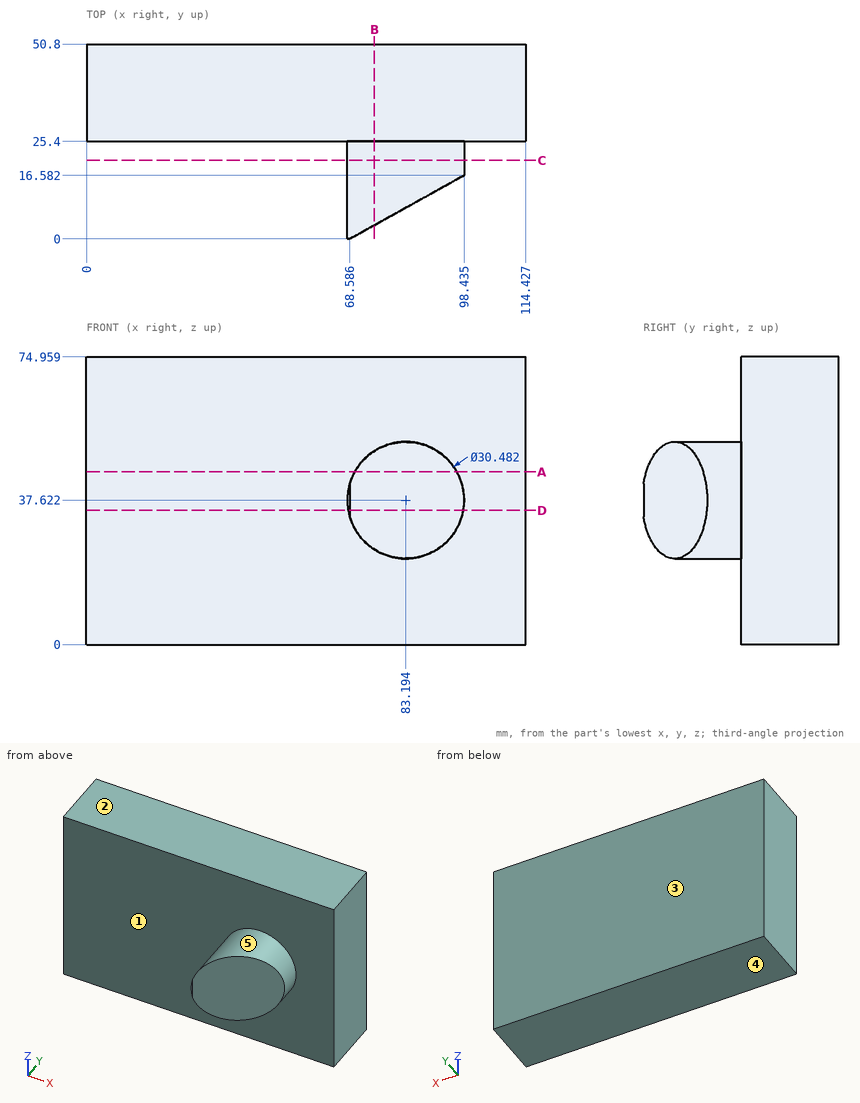
For this review, use the dimensioned drawing (mm, ordinates from the lowest corner) and the shaded views. A direction names the side the tool comes from. Round coordinates to 2 decimals unless told otherwise and drop trailing zeros. Order: outer loops, then holes, each group sorted by start corner. A loop starts at its lowest first (then second) coordinate and runs counter-clockwise, first axis right, second up. Notation, with made-up numbers: (-28, 58.5) -> (5, 58.5) arc R18 cw to (5, 80.5) -> close; hole circle Ø8 at (-0.75, 5). An arc over 180 degrees is marked (long way). Put each result on its own line as item: value.
Q1. Mouldability with a two-part tool opening along Y and no side actions: class the marked faces 1, 2 and 3 as pulls with the +Y half, pulls with the -Y half, needs draft (parallel to the pull), parting line crosses it, or undercut.
Check result:
face 1: pulls with the -Y half
face 2: needs draft
face 3: pulls with the +Y half
Q2. Insertion check: pin 1 Ø12 at (x, y) = (64.5, 10.5) entering from -Z (1 decimal); pin 2 Ø1.5 at (x, y) = (102, 26.5) entering from -Z; pin 3 Ø2 at (x, y) = (86, 21.5) entering from +Z (1 decimal); pin 4 Ø2 at (y, z) = (9.5, 23) entering from +X (1 decimal). Each pin has a flat end and moves straight along its axis. Give the tip position at first contact, or say it passes through.
Check result:
pin 1: z = 29.2
pin 2: z = 0
pin 3: z = 52.8
pin 4: x = 87.5
Q3. Add section A-A on z = 45. Write out the cut boundary in (x, y) (1 decimal).
Check result:
outline: (0, 25.4) -> (69.9, 25.4) -> (69.9, 0.7) -> (96.5, 15.5) -> (96.5, 25.4) -> (114.4, 25.4) -> (114.4, 50.8) -> (0, 50.8) -> close
Q4. Add section D-D on z = 35. Write out the cut boundary in (x, y).
Check result:
outline: (0, 25.4) -> (68.18, 25.4) -> (68.18, 0) -> (68.59, 0) -> (98.21, 16.46) -> (98.21, 25.4) -> (114.43, 25.4) -> (114.43, 50.8) -> (0, 50.8) -> close
Q5. Add section C-C on y = 20.5. Write out the cut boundary in (x, z) (1 decimal), plus the area to 3 significant figures.
Check result:
outline: circle Ø30.5 at (83.2, 37.6)
area: 730 mm2
Q6. Add section B-B on x = 75. Write out the cut boundary in (y, z), plus the area to 4 significant figures.
Check result:
outline: (3.56, 24.77) -> (25.4, 24.77) -> (25.4, 0) -> (50.8, 0) -> (50.8, 74.96) -> (25.4, 74.96) -> (25.4, 50.47) -> (3.56, 50.47) -> close
area: 2,465 mm2
Q7. For probe 1 along Y at (x, z) = (86, 9); probe 2 along X at (y, z) = (23, 46) (1 decimal); probe 3 along X at (y, z) = (12, 33) (1 decimal), list the stretches that pass through material, from the lowest coordinate up. Write a range as [from, to].
Check result:
probe 1: [25.4, 50.8]
probe 2: [70.5, 95.9]
probe 3: [68.7, 90.2]
Q8. Machinability: for the marked faces 4 and 5, which of the approach directions +Z, -Z, +X, -X, +Y, -Y give a long, thin tool a straight path to every point of the face, cutting with its end or side? Answer none if there is none.
Check result:
face 4: -Z, +X, -X, +Y, -Y
face 5: -Y
